Autodesk Inventor part; units mm, degrees
ref_plane "YZ Plane" through (0, 0, 0) normal (1, 0, 0) x (0, 1, 0)
ref_plane "XZ Plane" through (0, 0, 0) normal (0, 1, 0) x (-1, 0, 0)
ref_plane "XY Plane" through (0, 0, 0) normal (0, 0, 1) x (1, 0, 0)
sketch "Sketch1" plane through (0, 0, 0) normal (0, 0, 1) x (1, 0, 0)
  circle A0 centre (0, 0) radius 8.5
  circle A1 centre (0, 0) radius 3.075
  circle A2 centre (0, 0) radius 0.75
  line L0 (0, 0) -> (-3.6062, -3.6062) construction
  line L1 (0, 0) -> (5.1, 0) construction
  line L2 (0, 0) -> (3.6062, 3.6062) construction
  line L3 (0, 0) -> (5.1, 0) construction
  circle A3 centre (-3.6062, -3.6062) radius 1
  circle A4 centre (3.6216, 3.6216) radius 1
  dimension "d0" = 17
  dimension "d1" = 6.15
  dimension "d2" = 1.5
  dimension "d3" = 5.1
  dimension "d4" = 135
  dimension "d5" = 5.1
  dimension "d6" = 45
  dimension "d7" = 2
  dimension "d8" = 2
extrude "Extrusion1" add sketch "Sketch1" along normal blind 3 contours A0 | A1 | A2
ref_plane "Work Plane1" through (-7.1967, -146.8933, 23.5) normal (1, 0, 0) x (0, 1, 0)
sketch "Sketch2" plane through (-7.1967, -146.8933, 23.5) normal (1, 0, 0) x (0, 1, 0)
  line L0 (146.8933, -23.5) -> (146.8933, 3.1)
  line L1 (146.8933, -23.5) -> (173.4933, -23.5) construction
  line L2 (146.8933, 3.1) -> (141.8933, 3.1)
  line L3 (146.8933, 3.1) -> (151.8933, 3.1) construction
  dimension "d11" = 26.6
  dimension "d12" = 90
  dimension "d13" = 5
  dimension "d14" = 180
ref_plane "Work Plane4" through (0, 0, 26.6) normal (0, 0, -1) x (-1, 0, 0)
extrude "Extrusion2" add sketch "Sketch1" along normal up to surface (23.6 mm away) from surface at 3 contours A0 | A1 | A2 | A3 | A4
extrude "Extrusion3" add sketch "Sketch1" against normal blind 1.65 contours A1 | A2
extrude "Extrusion4" add sketch "Sketch1" against normal blind 4.05 contours A2
equation "\"d5\" = d3"
equation "\"d8\" = d7"
properties part number "MOTOR"
Verification items for the finished model (mm, model axes). A direction names the side the tool comes from. Coordinates: 2 decimals unless noted, no trailing zeros. Loops run counter-clockwise (first coordinate to the right, second up) from the corner with the lowest first, then second, coordinate; pieces in that order, holes last. Notation, with made-up numbers: (24, 69) - (76, 69) arc R18 ccw to (76, 88) - close; hole circle Ø1 at (47.5, 75.5). An arc over 180 degrees is marked (long way). Return JSON: item names as keys, results as strings.
1. Tool access check on faces 4 (the cylindrical face through (4.57, -7.167, 13.114)), 5 (the flat face through (4, 0, 0)). Record the directions out of +Z, -Z, +X, -X, +Y, -Y that give a thin tool (end or side, any length) a straight path to the whole face; none if there is none.
Established:
{"face 4": "+Z, -Z", "face 5": "-Z"}
2. Section check A-A, the plane x = 0. Record the boundary of the cut face in (y, z) (3 decimals), then the cut area to 3 significant figures.
Established:
{"outline": "(-8.5, 0) - (-3.075, 0) - (-3.075, -1.65) - (-0.75, -1.65) - (-0.75, -4.05) - (0.75, -4.05) - (0.75, -1.65) - (3.075, -1.65) - (3.075, 0) - (8.5, 0) - (8.5, 26.6) - (-8.5, 26.6) - close", "area": "466 mm2"}
3. Section check C-C, the plane z = -1. Record the boundary of the cut face in (x, y) (3 decimals), then the cut area to 3 significant figures.
Established:
{"outline": "circle Ø6.15 at (0, 0)", "area": "29.7 mm2"}
4. Go/stop test with flat-tipped pins: pin 1 (4 mm diameter, centred on y = -6.5, z = 20.5, fed in from +X); pin 2 (2 mm diameter, centred on x = 4, y = 3, fed in from -Z); pin 3 (5 mm diameter, centred on x = -5, z = 15.5, fed in from -Y). Record where each tip stops, or that it passes through.
Established:
{"pin 1": "stops at x = 7.21", "pin 2": "stops at z = 0", "pin 3": "stops at y = -8.12"}
5. Thickness scan on L1, parallel to Z at x = -2, y = -3.75; L2, parallel to X at y = 6.5, z = 17.5; L3, parallel to X at y = 3.75, z = 2. Record the ranges inside material, lowest first.
Established:
{"L1": "z = 0 to 26.6", "L2": "x = -5.48 to 5.48", "L3": "x = -7.63 to 2.63, 4.61 to 7.63"}
6. Mould release check, pull along Y, two halves, no side actions. Record for faces 1 (the flat face through (-4, -4, 3)), 2 (the flat face through (0, 0, 26.6)), 3 (the cylindrical face through (-0.75, 0.03, -2.83)): +Y half, -Y half, draft (parallel to the pull), parting line (faces both ways), or undercut.
Established:
{"face 1": "undercut", "face 2": "draft", "face 3": "parting line"}
7. Section check D-D, the plane y = -7.5. Record the boundary of the cut face in (x, z), then the cut area to 3 significant figures.
Established:
{"outline": "(-4, 0) - (4, 0) - (4, 26.6) - (-4, 26.6) - close", "area": "213 mm2"}
